Autodesk Fusion 360 part; units mm, degrees
sketch "Sketch1" plane through (0, 0, 0) normal (0, 0, 1) x (1, 0, 0)
  circle A0 centre (0, 0) radius 25.4
  line L0 (-0.4775, -1.5) -> (-2.5981, -1.5)
  line L1 (0.4974, -1.5) -> (2.5981, -1.5)
  line L2 (-0.4775, -1.5) -> (-0.4775, -2.9618)
  line L3 (0.4974, -1.5) -> (0.4974, -2.9585)
  arc A1 (-0.4775, -2.9618) -> (0.4974, -2.9585) centre (0, 0) ccw
  arc A2 (2.5981, -1.5) -> (-2.5981, -1.5) centre (0, 0) ccw
  dimension "d1" = 6
  dimension "d2" = 50.8
extrude "Extrude1" add sketch "Sketch1" along normal blind 5
sketch "Sketch2" plane through (0, 0, 5) normal (0, 0, 1) x (-1, 0, 0)
  line L0 (-2.5981, 1.5) -> (-0.4974, 1.5)
  line L1 (-0.4974, 1.5) -> (-0.4974, 2.9585)
  arc A0 (0.4775, 2.9618) -> (-0.4974, 2.9585) centre (0, 0) ccw
  line L2 (0.4775, 2.9618) -> (0.4775, 1.5)
  line L3 (0.4775, 1.5) -> (2.5981, 1.5)
  arc A1 (-2.5981, 1.5) -> (2.5981, 1.5) centre (0, 0) ccw
  circle A2 centre (0, 0) radius 25.4
  circle A3 centre (0, 0) radius 8
  dimension "d6" = 16
extrude "Extrude2" cut sketch "Sketch2" against normal blind 3 contours A3
sketch "Sketch3" plane through (0, 0, 5) normal (0, 0, 1) x (-1, 0, 0)
  circle A0 centre (0, 0) radius 8
  circle A1 centre (0, 0) radius 25.4
  circle A2 centre (0, 0) radius 12.3693
  circle A3 centre (0, 0) radius 20.6155
  line L0 (12.3686, 0.1302) -> (20.6151, 0.1302)
  line L1 (7.7191, -9.6651) -> (13.7003, -15.4046)
  line L2 (-0.1309, -12.3686) -> (-0.1309, -20.6151)
  line L3 (-12.3686, 0.1298) -> (-20.6151, 0.1298)
  line L4 (0, 12.3693) -> (0, 20.6155)
  line L5 (8.5619, 8.9272) -> (13.7135, 15.3929)
  line L6 (-9.5501, 7.861) -> (-16, 13)
  line L7 (-8.971, -8.5159) -> (-14.1393, -15.0026)
extrude "Extrude3" cut sketch "Sketch3" against normal blind 5 contours A2 A3 L0 L5 | A2 A3 L1 L2 | A2 A3 L4 L6 | A2 A3 L3 L7
The listing builds one solid part. Answer for the finished solid, in the listing's coordinates (mm). Give positions to 0.01 mm unless a question says otherwise; leave off trailing zeros. Loops run counter-clockwise (first coordinate to the right, second up) from the corner with the lowest first, then second, coordinate; pieces in that order, holes last. Notation, with made-up numbers: M -28.5,5 L -0.5,5 A21 ccw -0.5,35 Z; hole C -21,75 d5. An arc over 180 degrees is marked long. One line per item, written item: value.
Q1. A cutting plane is placed at D-D on y = -19. Determine the outline of the cut face in (x, z), then the cut area to 3 significant figures.
Working result:
outline: M -16.86,0 L 0,0 L 0,5 L -16.86,5 Z; M 8,0 L 16.86,0 L 16.86,5 L 8,5 Z
area: 129 mm^2
Q2. Flat-ended cylindrical pins translate along their axes: P1, Ø2.5, axis at x = -15, z = 3, coming from the -Y side; P2, Ø14.5, axis at x = 0, y = 0, coming from the +Z side; P3, Ø1.5, axis at x = 17.5, z = 1.5, coming from the +Y side. Find the tip coordinate at first contact, or state that the pin passes through.
Working result:
P1: stops at y = -21.36
P2: stops at z = 2
P3: stops at y = 19.09
Q3. A cutting plane is placed at B-B on x = -9.5. Determine the outline of the cut face in (y, z), then the cut area to 3 significant figures.
Working result:
outline: M -23.56,0 L -10.1,0 L -10.1,5 L -23.56,5 Z; M -7.92,0 L 11.37,0 L 11.37,5 L -7.92,5 Z; M 18.3,0 L 23.56,0 L 23.56,5 L 18.3,5 Z
area: 190 mm^2
Q4. A cutting plane is placed at A-A on y = -6.5. Determine the outline of the cut face in (x, z).
Working result:
outline: M -24.55,0 L -19.56,0 L -19.56,5 L -24.55,5 Z; M -10.52,0 L 24.55,0 L 24.55,5 L 4.66,5 L 4.66,2 L -4.66,2 L -4.66,5 L -10.52,5 Z
Q5. A cutting plane is placed at C-C on z = 1.4. Determine the outline of the cut face in (x, y), then the cut area to 3 significant figures.
Working result:
outline: C 0,0 d50.8; hole M -20.62,-0.13 A20.62 ccw -13.71,-15.39 L -8.56,-8.93 A12.37 cw -12.37,-0.13 Z; hole M -13.7,15.4 L -7.72,9.67 A12.37 cw 0.13,12.37 L 0.13,20.62 A20.62 ccw Z; hole M -2.6,-1.5 L -0.48,-1.5 L -0.48,-2.96 A3 ccw 0.5,-2.96 L 0.5,-1.5 L 2.6,-1.5 A3 ccw long Z; hole M 0,-20.62 A20.62 ccw 16,-13 L 9.55,-7.86 A12.37 cw 0,-12.37 Z; hole M 8.97,8.52 A12.37 cw 12.37,-0.13 L 20.62,-0.13 A20.62 ccw 14.14,15 Z
area: 1,560 mm^2
Q6. Find the intervals of material crossed by line 1 (Y direction, x = -11, z = 3.2); line 2 (X direction, y = 3.5, z = 3.7); line 3 (Z direction, x = -0.5, y = -5.5), in increasing order. Write a range as from..to.
Working result:
line 1: y = -22.89..-11.99, -5.66..12.81, 17.44..22.89
line 2: x = -25.16..-7.19, 7.19..11.86, 20.32..25.16
line 3: z = 0..2
Q7. Determine the mould class of faces 1 (the face through (-0.478, -2, 1)), 2 (the face through (-5.506, 24.796, 2.465)), 3 (the face through (-11.1, -12.11, 2.54)), 4 (the face through (0, -5, 0)) for opening direction X: +X half, -X half, draft (parallel to the pull), parting line (faces both ways), or undercut.
Working result:
face 1: undercut
face 2: parting line
face 3: undercut
face 4: draft
